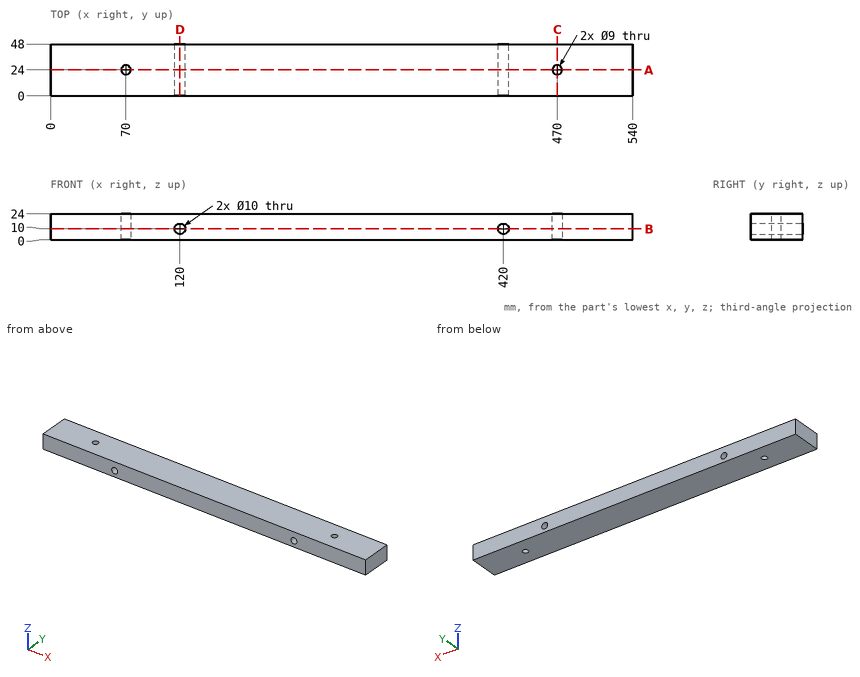
Source: three-view drawing plus pictorial views. Frame: mm from the lowest corner of the part. Round coordinates to 2 decimals unless told otherwise and drop trailing zeros. Write each loop counter-clockwise with the first axis right and the second up, starting at its lowest first coordinate (ties: lowest second). Pieces come first, ordered by that corner, then holes. Notation, with made-up numbers: M 67,-36.5 L 74,-36.5 A6 cw 74,-29.5 Z; hole C 60.5,72 d8. An arc over 180 degrees is marked long. One line per item, written item: value. Start each with the question number.
Item 1: Section query C-C (x = 470). Return the cut outline in (y, z), plus the area to 3 significant figures.
Item 2: Section query D-D (x = 120). Return the cut outline in (y, z), plus the area to 3 significant figures.
Item 3: Ray query, L1, parallel to X at y = 25.5, z = 21.5; L2, parallel to Y at x = 470, z = 12.5; L3, parallel to Z at x = 120, y = 36.5. Return the intervals inside material, ascending. Write a range as from..to.
Item 4: Section query A-A (y = 24). Return the cut outline in (x, z), plus the area to 3 significant figures.
Item 5: Pin query (flat end, axial travel): pin 1 (9 mm diameter, centred on x = 420, z = 10, fed in from -Y). Return the tip coordinate at first contact, or that it passes through.
Item 6: Section query B-B (z = 10). Return the cut outline in (x, y).
Result set:
1. outline: M 0,0 L 19.5,0 L 19.5,24 L 0,24 Z; M 28.5,0 L 48,0 L 48,24 L 28.5,24 Z
1. area: 936 mm²
2. outline: M 0,0 L 48,0 L 48,5 L 0,5 Z; M 0,15 L 48,15 L 48,24 L 0,24 Z
2. area: 672 mm²
3. L1: x = 0..65.76, 74.24..465.76, 474.24..540
3. L2: y = 0..19.5, 28.5..48
3. L3: z = 0..5, 15..24
4. outline: M 0,0 L 65.5,0 L 65.5,24 L 0,24 Z; M 74.5,0 L 465.5,0 L 465.5,24 L 74.5,24 Z; M 474.5,0 L 540,0 L 540,24 L 474.5,24 Z; hole C 120,10 d10; hole C 420,10 d10
4. area: 12,400 mm²
5. pin 1: passes through
6. outline: M 0,0 L 115,0 L 115,48 L 0,48 Z; M 125,0 L 415,0 L 415,48 L 125,48 Z; M 425,0 L 540,0 L 540,48 L 425,48 Z; hole C 70,24 d9; hole C 470,24 d9
